Here's how the part is built. I have some questions about the finished solid (model axes, mm). Face numbers are marked on the shaded views. A direction names the side the tool comes from. Round coordinates to 2 decimals unless told otherwise and drop trailing zeros. Write each loop counter-clockwise with the first axis right and the second up, starting at its lowest first coordinate (ties: lowest second). Pieces come first, ordered by that corner, then holes. Notation, with made-up numbers: (86.25, 7) -> (131.25, 7) arc R23 ccw to (131.25, 41) -> close; hole circle Ø1 at (63, 21.5). An arc over 180 degrees is marked (long way). Answer as CSV lines item,"result".
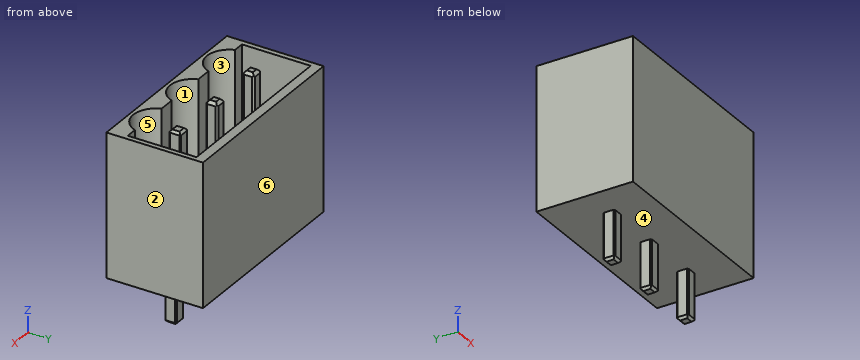
from build123d import *

# Parameters (mm, degrees)
SKETCH_1_W          = 16.4
SKETCH_1_H          = 8.2
EXTRUDE_1_DEPTH     = 12.1
SKETCH_4_R          = 1.25
CUT_EXTRUDE_3_DEPTH = 8
CUT_EXTRUDE_4_DEPTH = 7.8
SKETCH_7_W          = 1
SKETCH_7_H          = 1
EXTRUDE_2_DEPTH     = 8
CHAMFER_1_SIZE      = 0.15
CHAMFER_2_SIZE      = 0.25
SKETCH_8_W          = 1
SKETCH_8_H          = 1
EXTRUDE_3_DEPTH     = 4
CHAMFER_6_SIZE      = 0.1
CHAMFER_7_SIZE      = 0.2
CHAMFER_10_SIZE     = 0.1
CHAMFER_11_SIZE     = 0.2


with BuildPart() as part:
    # Эскиз1 → Бобышка-Вытянуть1 (new body)
    with BuildSketch(Plane.XY):
        Rectangle(SKETCH_1_W, SKETCH_1_H)
    extrude(amount=EXTRUDE_1_DEPTH)

    # Эскиз4 → Вырез-Вытянуть3 (cut)
    with BuildSketch(Plane.XY.offset(12.1)):
        with Locations((-5, 0)):
            Circle(SKETCH_4_R)
        Circle(SKETCH_4_R)
        with Locations((5, 0)):
            Circle(SKETCH_4_R)
    extrude(amount=-CUT_EXTRUDE_3_DEPTH, mode=Mode.SUBTRACT)

    # Эскиз5 → Вырез-Вытянуть4 (cut)
    with BuildSketch(Plane.XY.offset(12.1)):
        with BuildLine():
            Line((-7.745621634, 0), (-7.745621634, 3.292901982))
            Line((-7.745621634, 3.292901982), (2.778509544, 3.292901982))
            Line((2.778509544, 3.292901982), (7.778509544, 3.292901982))
            Line((7.778509544, 3.292901982), (7.778509544, -2.548957219))
            Line((7.778509544, -2.548957219), (6.80582632, -2.548957219))
            ThreePointArc((6.80582632, -2.548957219), (5, -3.818893996), (3.19417368, -2.548957219))
            Line((3.19417368, -2.548957219), (1.80582632, -2.548957219))
            ThreePointArc((1.80582632, -2.548957219), (0, -3.818893996), (-1.80582632, -2.548957219))
            Line((-1.80582632, -2.548957219), (-3.19417368, -2.548957219))
            ThreePointArc((-3.19417368, -2.548957219), (-5, -3.818893996), (-6.80582632, -2.548957219))
            Line((-6.80582632, -2.548957219), (-7.745621634, -2.548957219))
            Line((-7.745621634, -2.548957219), (-7.745621634, 0))
        make_face()
    extrude(amount=-CUT_EXTRUDE_4_DEPTH, mode=Mode.SUBTRACT)

    # Эскиз7 → Бобышка-Вытянуть2 (add)
    with BuildSketch(Plane.XY.offset(4.1)):
        Rectangle(SKETCH_7_W, SKETCH_7_H)
        with Locations((-5, 0)):
            Rectangle(SKETCH_7_W, SKETCH_7_H)
        with Locations((5, 0)):
            Rectangle(SKETCH_7_W, SKETCH_7_H)
    extrude(amount=EXTRUDE_2_DEPTH)

    # Фаска1
    chamfer_1_edges = [part.edges().sort_by_distance(p)[0] for p in [
        (-4.5, -0.5, 8.1),
        (-4.5, 0.5, 8.1),
        (-5.5, 0.5, 8.1),
        (-5.5, -0.5, 8.1),
        (0.5, -0.5, 8.1),
        (0.5, 0.5, 8.1),
        (-0.5, 0.5, 8.1),
        (-0.5, -0.5, 8.1),
    ]]
    chamfer(chamfer_1_edges, length=CHAMFER_1_SIZE)

    # Фаска2
    # the kernel refuses this chamfer: 0.25 mm, written as the material it takes off along each edge
    with BuildSketch(Plane(origin=(-0.5, -0.992920747, 12.1), x_dir=(-0.027495876610586414, 0, -0.9996219169112968), z_dir=(0, 1, 0)), Plane(origin=(-0.992920747, 0.5, 12.1), x_dir=(0, 0.027495876610586414, -0.9996219169112968), z_dir=(1, 0, 0)), Plane(origin=(0.5, 0.992920747, 12.1), x_dir=(0.027495876610586414, 0, -0.9996219169112968), z_dir=(0, -1, 0)), Plane(origin=(0.992920747, -0.5, 12.1), x_dir=(0, -0.027495876610586414, -0.9996219169112968), z_dir=(-1, 0, 0)), Plane(origin=(-4.5, 0.992920747, 12.1), x_dir=(0.02749587661058555, 0, -0.9996219169112968), z_dir=(0, -1, 0)), Plane(origin=(-4.007079253, -0.5, 12.1), x_dir=(0, -0.027495876610586414, -0.9996219169112968), z_dir=(-1, 0, 0)), Plane(origin=(-5.5, -0.992920747, 12.1), x_dir=(-0.02749587661058555, 0, -0.9996219169112968), z_dir=(0, 1, 0)), Plane(origin=(-5.992920747, 0.5, 12.1), x_dir=(0, 0.027495876610586414, -0.9996219169112968), z_dir=(1, 0, 0))) as chamfer_2_piece_1:
        Polygon((CHAMFER_2_SIZE * 0.999621916911, -CHAMFER_2_SIZE * 0.0274958766106), (-CHAMFER_2_SIZE * 0.0274958766106, -CHAMFER_2_SIZE * 0.999621916911), (0, 0), align=None)
    extrude(amount=1.985841494, mode=Mode.SUBTRACT)

    # Эскиз8 → Бобышка-Вытянуть3 (add)
    with BuildSketch(Plane(origin=(0, -4.1, 0), x_dir=(-1, 0, 0), z_dir=(0, 0, 1))):
        with Locations((0, -3.75)):
            Rectangle(SKETCH_8_W, SKETCH_8_H)
        with Locations((5, -3.75)):
            Rectangle(SKETCH_8_W, SKETCH_8_H)
        with Locations((-5, -3.75)):
            Rectangle(SKETCH_8_W, SKETCH_8_H)
    extrude(amount=-EXTRUDE_3_DEPTH)

    # Фаска6
    chamfer_6_edges = [part.edges().sort_by_distance(p)[0] for p in [
        (5.5, -0.5, 8.1),
        (5.5, 0.5, 8.1),
        (4.5, 0.5, 8.1),
        (4.5, -0.5, 8.1),
    ]]
    chamfer(chamfer_6_edges, length=CHAMFER_6_SIZE)

    # Фаска7
    # the kernel refuses this chamfer: 0.2 mm, written as the material it takes off along each edge
    with BuildSketch(Plane(origin=(5.5, 0.914336598, 12.1), x_dir=(0.02749587661058742, 0, -0.9996219169112966), z_dir=(0, -1, 0)), Plane(origin=(5.914336598, -0.5, 12.1), x_dir=(0, -0.02749587661058634, -0.9996219169112966), z_dir=(-1, 0, 0)), Plane(origin=(4.5, -0.914336598, 12.1), x_dir=(-0.02749587661058742, 0, -0.9996219169112966), z_dir=(0, 1, 0)), Plane(origin=(4.085663402, 0.5, 12.1), x_dir=(0, 0.02749587661058634, -0.9996219169112966), z_dir=(1, 0, 0))) as chamfer_7_piece_1:
        Polygon((CHAMFER_7_SIZE * 0.999621916911, -CHAMFER_7_SIZE * 0.0274958766106), (-CHAMFER_7_SIZE * 0.0274958766106, -CHAMFER_7_SIZE * 0.999621916911), (0, 0), align=None)
    extrude(amount=1.828673195, mode=Mode.SUBTRACT)

    # Фаска10
    chamfer_10_edges = [part.edges().sort_by_distance(p)[0] for p in [
        (-4.5, 0.15, -2),
        (-4.5, -0.85, -2),
        (-5.5, -0.85, -2),
        (-5.5, 0.15, -2),
        (0.5, 0.15, -2),
        (0.5, -0.85, -2),
        (-0.5, -0.85, -2),
        (-0.5, 0.15, -2),
        (5.5, 0.15, -2),
        (5.5, -0.85, -2),
        (4.5, -0.85, -2),
        (4.5, 0.15, -2),
    ]]
    chamfer(chamfer_10_edges, length=CHAMFER_10_SIZE)

    # Фаска11
    # the kernel refuses this chamfer: 0.2 mm, written as the material it takes off along each edge
    with BuildSketch(Plane(origin=(-4.5, 0.564336598, -4), x_dir=(0.027495876610587302, 0, 0.9996219169112966), z_dir=(0, -1, 0)), Plane(origin=(-5.914336598, 0.15, -4), x_dir=(0, 0.027495876610586355, 0.9996219169112966), z_dir=(1, 0, 0)), Plane(origin=(-5.5, -1.264336598, -4), x_dir=(-0.027495876610587302, 0, 0.9996219169112966), z_dir=(0, 1, 0)), Plane(origin=(-4.085663402, -0.85, -4), x_dir=(0, -0.027495876610586223, 0.9996219169112966), z_dir=(-1, 0, 0)), Plane(origin=(0.914336598, -0.85, -4), x_dir=(0, -0.027495876610586223, 0.9996219169112966), z_dir=(-1, 0, 0)), Plane(origin=(-0.5, -1.264336598, -4), x_dir=(-0.027495876610586223, 0, 0.9996219169112966), z_dir=(0, 1, 0)), Plane(origin=(-0.914336598, 0.15, -4), x_dir=(0, 0.027495876610586355, 0.9996219169112966), z_dir=(1, 0, 0)), Plane(origin=(0.5, 0.564336598, -4), x_dir=(0.027495876610586223, 0, 0.9996219169112966), z_dir=(0, -1, 0)), Plane(origin=(4.5, -1.264336598, -4), x_dir=(-0.027495876610587302, 0, 0.9996219169112966), z_dir=(0, 1, 0)), Plane(origin=(4.085663402, 0.15, -4), x_dir=(0, 0.027495876610586355, 0.9996219169112966), z_dir=(1, 0, 0)), Plane(origin=(5.5, 0.564336598, -4), x_dir=(0.027495876610587302, 0, 0.9996219169112966), z_dir=(0, -1, 0)), Plane(origin=(5.914336598, -0.85, -4), x_dir=(0, -0.027495876610586223, 0.9996219169112966), z_dir=(-1, 0, 0))) as chamfer_11_piece_1:
        Polygon((CHAMFER_11_SIZE * 0.999621916911, CHAMFER_11_SIZE * 0.0274958766106), (-CHAMFER_11_SIZE * 0.0274958766106, CHAMFER_11_SIZE * 0.999621916911), (0, 0), align=None)
    extrude(amount=1.828673195, mode=Mode.SUBTRACT)


solid = part.part
Item 1: Suppose I cut it at A-A, the plane y = 0.75. List the corners of the cut face in (x, z) for me, then the cut area to 3 significant figures.
Results found:
outline,"(-8.2, 0) -> (8.2, 0) -> (8.2, 12.1) -> (7.78, 12.1) -> (7.78, 4.3) -> (6, 4.3) -> (6, 4.1) -> (4, 4.1) -> (4, 4.3) -> (1, 4.3) -> (1, 4.1) -> (-1, 4.1) -> (-1, 4.3) -> (-4, 4.3) -> (-4, 4.1) -> (-6, 4.1) -> (-6, 4.3) -> (-7.75, 4.3) -> (-7.75, 12.1) -> (-8.2, 12.1) -> close"
area,"76.2 mm²"
Item 2: For the marked faces 1 and 2, which set-ups out of +Z, -Z, +X, -X, +Y, -Y let a thin tool reach every point of the face, with its end or its side?
Results found:
face 1,"+Z"
face 2,"+Z, -Z, +X, +Y, -Y"
Item 3: Suppose I cut it at D-D, the plane x = 0. List the corners of the cut face in (y, z) for me, then the cut area to 3 significant figures.
Results found:
outline,"(-4.1, 0) -> (-0.85, 0) -> (-0.85, -3.8) -> (-0.65, -4) -> (-0.05, -4) -> (0.15, -3.8) -> (0.15, 0) -> (4.1, 0) -> (4.1, 12.1) -> (3.29, 12.1) -> (3.29, 4.3) -> (1.25, 4.3) -> (1.25, 4.1) -> (0.5, 4.1) -> (0.5, 11.85) -> (0.25, 12.1) -> (-0.25, 12.1) -> (-0.5, 11.85) -> (-0.5, 4.1) -> (-1.25, 4.1) -> (-1.25, 4.3) -> (-3.82, 4.3) -> (-3.82, 12.1) -> (-4.1, 12.1) -> close"
area,"55.1 mm²"
Item 4: Suppose I cut it at B-B, the plane x = 5. List the corners of the cut face in (y, z) for me, then the cut area to 3 significant figures.
Results found:
outline,"(-4.1, 0) -> (-0.85, 0) -> (-0.85, -3.8) -> (-0.65, -4) -> (-0.05, -4) -> (0.15, -3.8) -> (0.15, 0) -> (4.1, 0) -> (4.1, 12.1) -> (3.29, 12.1) -> (3.29, 4.3) -> (1.25, 4.3) -> (1.25, 4.1) -> (0.5, 4.1) -> (0.5, 11.9) -> (0.3, 12.1) -> (-0.3, 12.1) -> (-0.5, 11.9) -> (-0.5, 4.1) -> (-1.25, 4.1) -> (-1.25, 4.3) -> (-3.82, 4.3) -> (-3.82, 12.1) -> (-4.1, 12.1) -> close"
area,"55.2 mm²"
Item 5: Suppose I cut it at C-C, the plane z = 7.5. State how many separate pieces and enclosed holes the cut face has, then the cut area to 3 significant figures.
Results found:
separate pieces,"4"
enclosed holes,"1"
area,"36.7 mm²"
Item 6: If we mould it in two halves opening along Y, with no side actions, what happens to the marked faces 3, 4, 5 and 6? For each: pulls with the +Y half, pulls with the -Y half, needs draft (parallel to the pull), parting line crosses it, or undercut.
Results found:
face 3,"undercut"
face 4,"needs draft"
face 5,"undercut"
face 6,"pulls with the +Y half"
Item 7: Will these pins go through, and if not, where does the flat tip stop? pin 1 (1.5 mm diameter, centred on x = -4, y = -0.5, fed in from -Z); pin 2 (0.9 mm diameter, centred on x = 5, z = -1.5, fed in from -Y); pin 3 (0.6 mm diameter, centred on x = 0, z = -2, fed in from +Y).
Results found:
pin 1,"stops at z = -4"
pin 2,"stops at y = -0.85"
pin 3,"stops at y = 0.15"
Item 8: I need wall thicknesses on L1, parallel to X at y = 0.25, z = 4.75; L2, parallel to Y at x = 0, z = 4.25; L3, parallel to X at y = 1.75, z = 11.5. Which ranges of each line are inside material? Lowest first, please.
Results found:
L1,"x = -8.2 to -7.75, -5.5 to -4.5, -0.5 to 0.5, 4.5 to 5.5, 7.78 to 8.2"
L2,"y = -4.1 to -1.25, -0.5 to 0.5, 1.25 to 4.1"
L3,"x = -8.2 to -7.75, 7.78 to 8.2"
